Design review of the part shown in the three views and the two pictorial views. Dimensions are in mm from the part's minimum x, y and z. A direction names the side the tool comes from. Coordinates: 2 decimals unless noted, no trailing zeros. Write each loop counter-clockwise with the first axis right and the second up, starting at its lowest first coordinate (ties: lowest second). Pieces come first, ordered by that corner, then holes. Notation, with made-up numbers: (46, 78) -> (101, 78) arc R34 cw to (101, 112) -> close; hole circle Ø2 at (37, 76). An arc over 180 degrees is marked (long way). Answer in a Markdown table with one row per item. Add a question column.
Item 1: Take a section at C-C, the plane z = 4. Write out the cut boundary in (x, y) (1 decimal).
Item 2: To check wall thickness, follow line 1 (X direction, y = 9.25, z = 7.75); line 2 (X direction, y = 14, z = 5.75); line 3 (Y direction, x = 9.5, z = 6) (1 decimal). State the ranges of each line that lie inside material, in increasing order.
Item 3: For the marked faces 5, 6 and 7, list the 3-axis set-ups (+Z, -Z, +X, -X, +Y, -Y) from which the entire face can be reached by the end or side of a thin tool; tool diameter is ignored.
Item 4: Take a section at B-B, the plane x = 28.5. Write out the cut boundary in (y, z) (1 decimal), and give its area (3 significant figures).
Item 5: Clearance check with flat-ended pins moving along their axes: P1, Ø3, axis at x = 18.5, z = 4.5, coming from the -Y side; P2, Ø3.5, axis at x = 3.5, y = 4, coming from the -Z side; P3, Ø3, axis at x = 31.89, y = 7.49, coming from the +Z side. State where each tip first meets the part, or that it passes through.
Item 6: Take a section at D-D, the plane y = 6.75. Write out the cut boundary in (x, z).
Item 7: Draft analysis for pull direction Y (two halves, no side actions). For the marked faces 1, 2, 3 and 4, state which applies: released by +Y, released by -Y, zero draft, split by the parting line, or undercut.
Item 8: Take a section at A-A, the plane y = 4.75. Write out the cut boundary in (x, z).
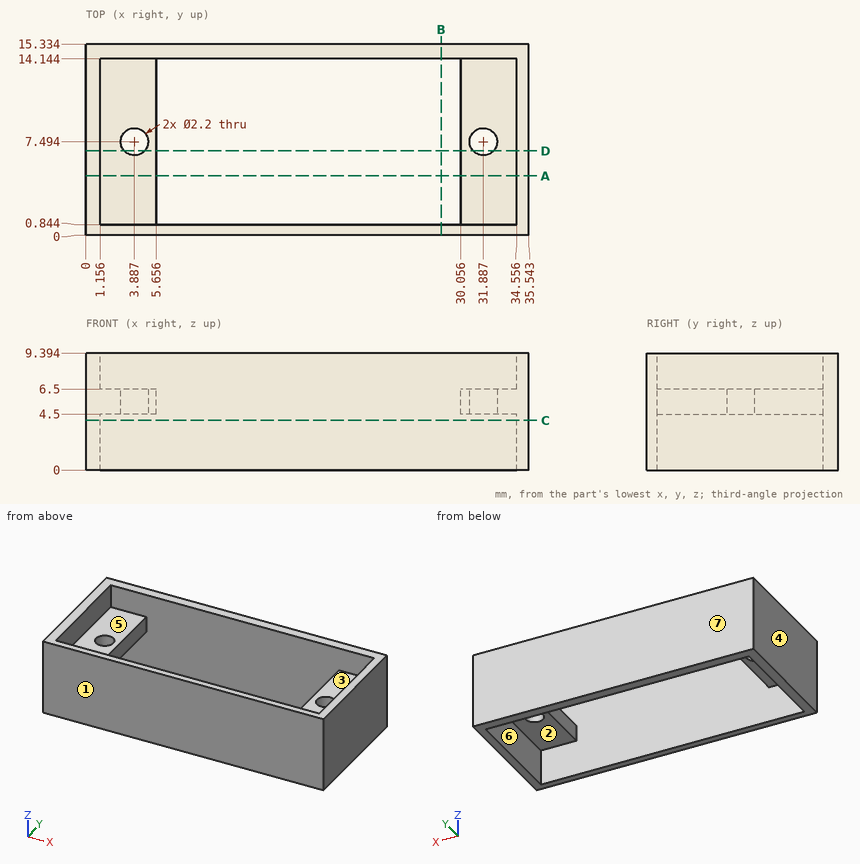
Answers:
| question | item | result |
|---|---|---|
| 1 | outline | (0, 0) -> (35.5, 0) -> (35.5, 15.3) -> (0, 15.3) -> close; hole (1.2, 0.8) -> (34.6, 0.8) -> (34.6, 14.1) -> (1.2, 14.1) -> close |
| 2 | line 1 | x = 0 to 1.16, 34.56 to 35.54 |
| 2 | line 2 | x = 0 to 5.66, 30.06 to 35.54 |
| 2 | line 3 | y = 0 to 0.8, 14.1 to 15.3 |
| 3 | face 5 | +Z |
| 3 | face 6 | -Z |
| 3 | face 7 | +Z, -Z, +X, -X, +Y |
| 4 | outline | (0, 0) -> (0.8, 0) -> (0.8, 9.4) -> (0, 9.4) -> close; (14.1, 0) -> (15.3, 0) -> (15.3, 9.4) -> (14.1, 9.4) -> close |
| 4 | area | 19.1 mm^2 |
| 5 | P1 | stops at y = 0 |
| 5 | P2 | stops at z = 4.5 |
| 5 | P3 | stops at z = 6.5 |
| 6 | outline | (0, 0) -> (1.16, 0) -> (1.16, 4.5) -> (3.08, 4.5) -> (3.08, 6.5) -> (1.16, 6.5) -> (1.16, 9.39) -> (0, 9.39) -> close; (4.7, 4.5) -> (5.66, 4.5) -> (5.66, 6.5) -> (4.7, 6.5) -> close; (30.06, 4.5) -> (31.08, 4.5) -> (31.08, 6.5) -> (30.06, 6.5) -> close; (32.7, 4.5) -> (34.56, 4.5) -> (34.56, 0) -> (35.54, 0) -> (35.54, 9.39) -> (34.56, 9.39) -> (34.56, 6.5) -> (32.7, 6.5) -> close |
| 7 | face 1 | released by -Y |
| 7 | face 2 | undercut |
| 7 | face 3 | undercut |
| 7 | face 4 | zero draft |
| 8 | outline | (0, 0) -> (1.16, 0) -> (1.16, 4.5) -> (5.66, 4.5) -> (5.66, 6.5) -> (1.16, 6.5) -> (1.16, 9.39) -> (0, 9.39) -> close; (30.06, 4.5) -> (34.56, 4.5) -> (34.56, 0) -> (35.54, 0) -> (35.54, 9.39) -> (34.56, 9.39) -> (34.56, 6.5) -> (30.06, 6.5) -> close |
